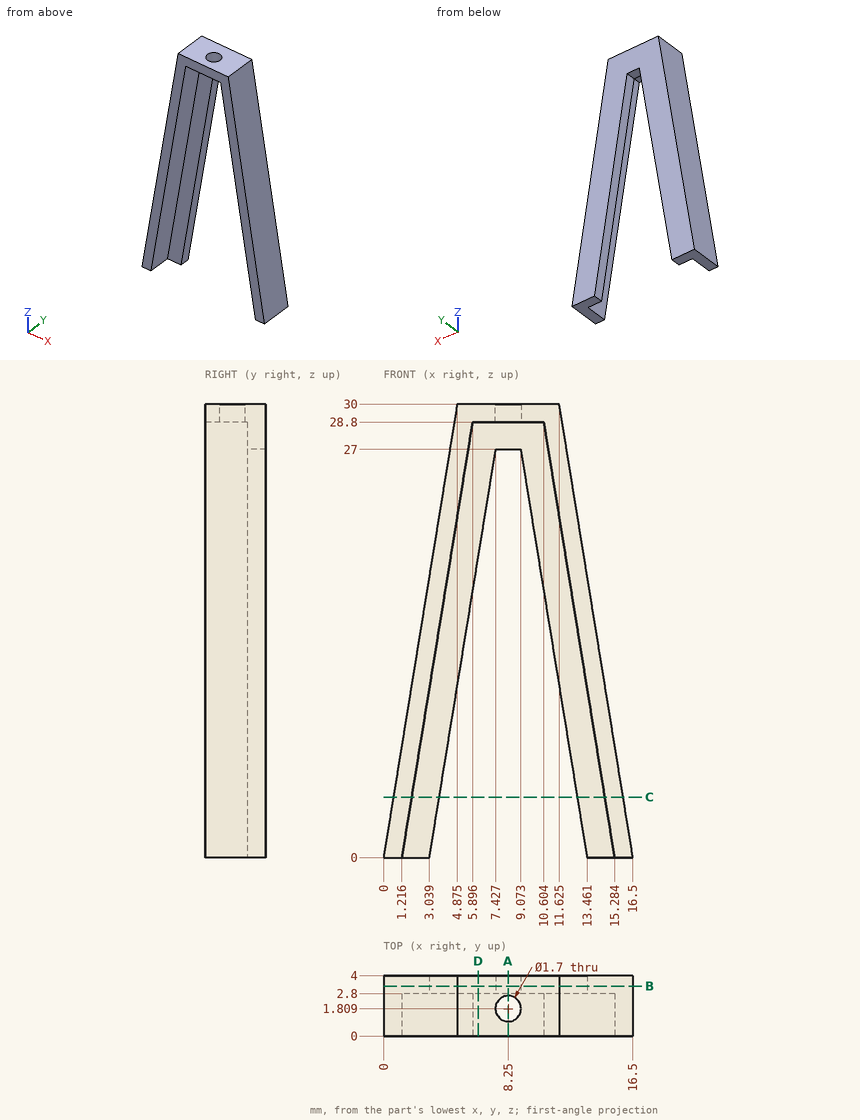
Study the drawing (mm; zero at the part's minimum x, y, z) and answer. Round coordinates to 2 decimals unless told otherwise and drop trailing zeros. Write each loop counter-clockwise with the first axis right and the second up, starting at its lowest first coordinate (ties: lowest second). Pieces come first, ordered by that corner, then holes.
1) A cutting plane is placed at D-D (x = 6.25). Give the vertices of the cut face in (y, z).
2) Straight lines are drawn through the part: line 1 (Y direction, x = 8.25, z = 29.25); line 2 (X direction, y = 0.7, z = 5.5); line 3 (X direction, y = 1.2, z = 1). For each, find the intervals that lie inside material, in ascending order.
3) A cutting plane is placed at A-A (x = 8.25). Give the vertices of the cut face in (y, z).
4) A cutting plane is placed at B-B (y = 3.3). Give the vertices of the cut face in (x, z) (1 decimal), plus the area to 3 significant figures.
5) A cutting plane is placed at C-C (z = 4). Give the vertices of the cut face in (x, y).
6) Given pin 1 Ø2 at (x, y) = (7.5, 1.5) entering from -Z; pin 2 Ø1.5 at (x, z) = (5, 11) entering from -Y; pin 3 Ø1.5 at (y, z) = (0.5, 6.5) entering from -X, each flat-ended and moving along its own axis, determine where each tip first touches the part or whether it passes through.
Completed:
1. outline: (0, 28.8) - (2.8, 28.8) - (2.8, 19.76) - (4, 19.76) - (4, 30) - (0, 30) - close
2. line 1: y = 0 to 0.96, 2.66 to 4
2. line 2: x = 0.89 to 2.11, 14.39 to 15.61
2. line 3: x = 0.16 to 1.38, 15.12 to 16.34
3. outline: (0, 28.8) - (0.96, 28.8) - (0.96, 30) - (0, 30) - close; (2.66, 28.8) - (2.8, 28.8) - (2.8, 27) - (4, 27) - (4, 30) - (2.66, 30) - close
4. outline: (0, 0) - (3, 0) - (7.4, 27) - (9.1, 27) - (13.5, 0) - (16.5, 0) - (11.6, 30) - (4.9, 30) - close
4. area: 186 mm2
5. outline: (0.65, 0) - (1.87, 0) - (1.87, 2.8) - (3.69, 2.8) - (3.69, 4) - (0.65, 4) - close; (12.81, 2.8) - (14.63, 2.8) - (14.63, 0) - (15.85, 0) - (15.85, 4) - (12.81, 4) - close
6. pin 1: stops at z = 28.8
6. pin 2: stops at y = 2.8
6. pin 3: stops at x = 0.93
